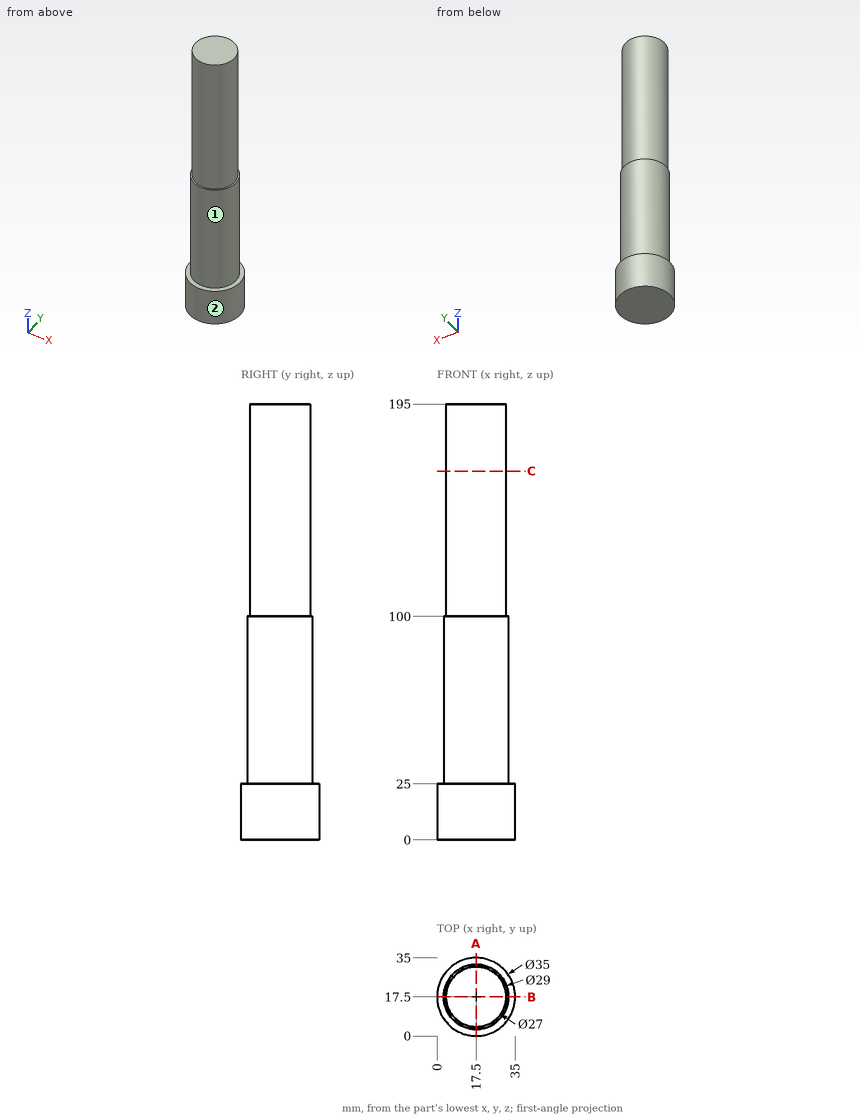
Here's the drawing with two shaded views (mm, measured from the low corner). I have some questions. A direction names the side the tool comes from. Give positions to 0.01 mm unless a question says otherwise; leave off trailing zeros. Order: outer loops, then holes, each group sorted by start corner. A loop starts at its lowest first (then second) coordinate and runs counter-clockwise, first axis right, second up. Notation, with made-up numbers: M -12.5,35 L 20.5,35 A17 cw 20.5,61 Z; hole C 67.25,-19.5 d3. An arc over 180 degrees is marked long. Answer as a JSON object with one key per item and string values. Group by question number.
1) Please list where these lines run through material, in increasing order: L1, parallel to Z at x = 29, y = 5; L2, parallel to Y at x = 16.5, z = 98; L3, parallel to Y at x = 17.5, z = 159.5. Write a range as [from, to].
2) Suppose I cut it at A-A, the plane x = 17.5. Write out the boundary of the cut face in (y, z).
3) Suppose I cut it at C-C, the plane z = 165. Write out the boundary of the cut face in (x, y), plus the area to 3 significant figures.
4) On a 3-axis mill with a long thin cutter (end or side, diameter ignored), from which of +Z, -Z, +X, -X, +Y, -Y can I reach the whole of each face in a straight line? I mean the marked faces 1 and 2. Say none if no direction works.
5) I'm going to push flat-ended pins straight in: pin 1 Ø1 at (y, z) = (21, 54.5) entering from -X; pin 2 Ø6 at (y, z) = (24.5, 169) entering from +X; pin 3 Ø1 at (x, z) = (17, 148) entering from -Y. Where does each tip first touch, or does it pass through?
Results found:
{
 "1": {"L1": "[0, 25]", "L2": "[3.03, 31.97]", "L3": "[4, 31]"},
 "2": {"outline": "M 0,0 L 35,0 L 35,25 L 32,25 L 32,100 L 31,100 L 31,195 L 4,195 L 4,100 L 3,100 L 3,25 L 0,25 Z"},
 "3": {"outline": "C 17.5,17.5 d27", "area": "573 mm²"},
 "4": {"face 1": "+Z", "face 2": "+Z, -Z"},
 "5": {"pin 1": "x = 3.31", "pin 2": "x = 30.39", "pin 3": "y = 4"}
}
